Read the model definition and answer for the solid it produces. Units are mm, in the model's axes. Give positions to 0.01 mm unless a question says otherwise; leave off trailing zeros. Order: outer loops, then holes, each group sorted by start corner. A loop starts at its lowest first (then second) coordinate and runs counter-clockwise, first axis right, second up. Notation, with made-up numbers: (27.5, 55) - (33.5, 55) arc R22 ccw to (33.5, 65) - close; hole circle Ø2 at (43, 83). An arc over 180 degrees is marked (long way). Write each question's results on one line, items separated by ' | '.
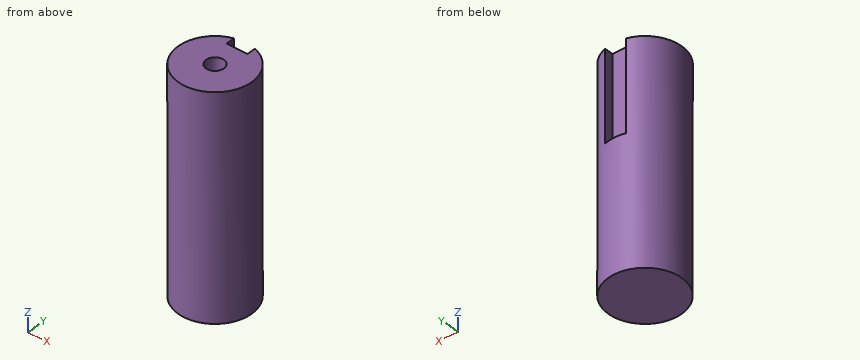
from build123d import *

# Parameters (mm, degrees)
ESQUISSE1_R             = 17.5
BOSS_EXTRU_1_DEPTH      = 105
ESQUISSE2_W             = 10
ESQUISSE2_H             = 7.08484742
ENL_V_MAT_EXTRU_1_DEPTH = 43
TROU_TARAUD_M101_D      = 8.5
TROU_TARAUD_M101_DEPTH  = 40
TROU_TARAUD_M101_TIP    = 2.553657631


with BuildPart() as part:
    # Esquisse1 → Boss.-Extru.1 (new body)
    with BuildSketch(Plane.XY):
        Circle(ESQUISSE1_R)
    extrude(amount=BOSS_EXTRU_1_DEPTH)

    # Esquisse2 → Enlèv. mat.-Extru.1 (cut)
    with BuildSketch(Plane.XY.offset(105)):
        with Locations((0, 16.04242371)):
            Rectangle(ESQUISSE2_W, ESQUISSE2_H)
    extrude(amount=-ENL_V_MAT_EXTRU_1_DEPTH, mode=Mode.SUBTRACT)

    # Trou taraudé M101
    with Locations(Plane.XY.offset(105)):
        with Locations((0, 0)):
            Hole(TROU_TARAUD_M101_D / 2, depth=TROU_TARAUD_M101_DEPTH)
            with Locations((0, 0, -(TROU_TARAUD_M101_DEPTH + TROU_TARAUD_M101_TIP / 2))):  # 118° drill point
                Cone(0, TROU_TARAUD_M101_D / 2, TROU_TARAUD_M101_TIP, mode=Mode.SUBTRACT)


solid = part.part
(1) Each of these flat-tipped pins is pushed along its axis until it touches: pin 1 (12 mm diameter, centred on x = 9.5, z = 40.5, fed in from +Y); pin 2 (1.3 mm diameter, centred on y = 15, z = 82.5, fed in from +X); pin 3 (4 mm diameter, centred on y = 6.5, z = 28.5, fed in from -X). Where does it stop, or does it pass through?
Conclusion:
pin 1: y = 17.15 | pin 2: x = 10.02 | pin 3: x = -16.91
(2) Section C-C (x = -6.5) is taken. Give the vertices of the cut face in (y, z), plus the area to 3 significant figures.
Conclusion:
outline: (-16.25, 0) - (16.25, 0) - (16.25, 105) - (-16.25, 105) - close | area: 3,410 mm^2
(3) Section B-B (y = 15) is taken. Give the vertices of the cut face in (x, z).
Conclusion:
outline: (-9.01, 0) - (9.01, 0) - (9.01, 105) - (5, 105) - (5, 62) - (-5, 62) - (-5, 105) - (-9.01, 105) - close
(4) Consider probe 1 along Y at (x, z) = (0, 73); probe 2 along X at (y, z) = (0, 82); probe 3 along X at (y, z) = (0.5, 61). Determine where each line is inside the solid, lowest interval first. Write a range as [from, to].
Conclusion:
probe 1: [-17.5, -4.25], [4.25, 12.5] | probe 2: [-17.5, -4.25], [4.25, 17.5] | probe 3: [-17.49, 17.49]
(5) Section A-A (z = 68.5) is taken. Give the vertices of the cut face in (x, y).
Conclusion:
outline: (-5, 12.5) - (-5, 16.77) arc R17.5 ccw (long way) to (5, 16.77) - (5, 12.5) - close; hole circle Ø8.5 at (0, 0)
(6) Section D-D (z = 41) is taken. Give the vertices of the cut face in (x, y), plus the area to 3 significant figures.
Conclusion:
outline: circle Ø35 at (0, 0) | area: 962 mm^2
